Build history of the part. All positions in model axes, mm. Face numbers are marked on the shaded views. A direction names the side the tool comes from. Give positions to 0.01 mm unless a question says otherwise; leave off trailing zeros. Write each loop counter-clockwise with the first axis right and the second up, starting at its lowest first coordinate (ties: lowest second). Pieces come first, ordered by that corner, then holes.
from build123d import *

# Parameters (mm, degrees)
SB_KIRI_80_X_6_1_DEPTH = 20


with BuildPart() as part:
    # Sketch1 → Sb kiriş 80 X 6(1) (new body)
    with BuildSketch(Plane.YZ):
        with BuildLine():
            Line((-20, -40), (-20, -38.04146021))
            ThreePointArc((-20, -38.04146021), (-19.289071417, -36.102349061), (-17.493231968, -35.082284273))
            Line((-17.493231968, -35.082284273), (-7.013536064, -33.335540874))
            ThreePointArc((-7.013536064, -33.335540874), (-3.421857166, -31.295411298), (-2, -27.417189))
            Line((-2, -27.417189), (-2, 27.417189))
            ThreePointArc((-2, 27.417189), (-3.421857166, 31.295411298), (-7.013536064, 33.335540874))
            Line((-7.013536064, 33.335540874), (-17.493231968, 35.082284273))
            ThreePointArc((-17.493231968, 35.082284273), (-19.289071417, 36.102349061), (-20, 38.04146021))
            Line((-20, 38.04146021), (-20, 40))
            Line((-20, 40), (20, 40))
            Line((20, 40), (20, 38.04146021))
            ThreePointArc((20, 38.04146021), (19.289071417, 36.102349061), (17.493231968, 35.082284273))
            Line((17.493231968, 35.082284273), (7.013536064, 33.335540874))
            ThreePointArc((7.013536064, 33.335540874), (3.421857166, 31.295411298), (2, 27.417189))
            Line((2, 27.417189), (2, -27.417189))
            ThreePointArc((2, -27.417189), (3.421857166, -31.295411298), (7.013536064, -33.335540874))
            Line((7.013536064, -33.335540874), (17.493231968, -35.082284273))
            ThreePointArc((17.493231968, -35.082284273), (19.289071417, -36.102349061), (20, -38.04146021))
            Line((20, -38.04146021), (20, -40))
            Line((20, -40), (-20, -40))
        make_face()
    extrude(amount=SB_KIRI_80_X_6_1_DEPTH)


solid = part.part
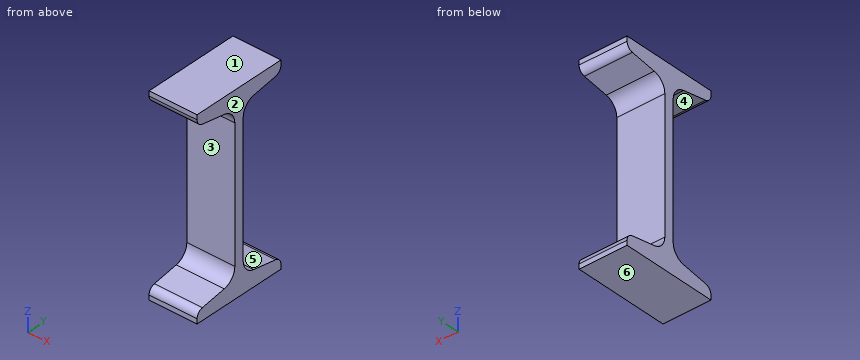
1. Saw through at C-C on y = -13.5. Give the cut face in (x, z).
2. Saw through at D-D on z = 2. Give the cut face in (x, y).
3. 3-axis set-ups, long thin cutter, end or side, ignore diameter. For the marked faces 4, 5 and 6: which of +Z, -Z, +X, -X, +Y, -Y reach the whole face in a straight line?
4. Drop flat-ended pins along their axis: pin 1 (12 mm diameter, centred on x = 7, z = 9, fed in from +Y); pin 2 (4 mm diameter, centred on x = 14.5, z = 30.5, fed in from +Y); pin 3 (6 mm diameter, centred on x = 11.5, z = 3, fed in from -Y). Give the stop position or say it passes through.
5. Saw through at B-B on x = 6.75. Give the cut face in (y, z).
6. Drill centre lines: line 1 along Y through (x, z) = (7.25, 12.5); line 2 along Z through (x, y) = (13.75, -5); line 3 along Z through (x, y) = (5, -10). Where is each one in solid material? Low to high.
7. Saw through at A-A on y = 5.5. Give the cut face in (x, z).
8. Mould opens along Z. For the marked faces 1, 2 and 3 say: pulls with the +Z half, pulls with the -Z half, needs draft (parallel to the pull), parting line crosses it, or undercut.
Outcome:
1. outline: (0, -40) - (20, -40) - (20, -34.42) - (0, -34.42) - close; (0, 34.42) - (20, 34.42) - (20, 40) - (0, 40) - close
2. outline: (0, -2) - (20, -2) - (20, 2) - (0, 2) - close
3. face 4: +X, -X, -Y
3. face 5: +X, -X, +Y
3. face 6: -Z, +X, -X, +Y, -Y
4. pin 1: stops at y = 2
4. pin 2: stops at y = 4.81
4. pin 3: stops at y = -2
5. outline: (-20, -40) - (20, -40) - (20, -38.04) arc R3 ccw to (17.49, -35.08) - (7.01, -33.34) arc R6 cw to (2, -27.42) - (2, 27.42) arc R6 cw to (7.01, 33.34) - (17.49, 35.08) arc R3 ccw to (20, 38.04) - (20, 40) - (-20, 40) - (-20, 38.04) arc R3 ccw to (-17.49, 35.08) - (-7.01, 33.34) arc R6 cw to (-2, 27.42) - (-2, -27.42) arc R6 cw to (-7.01, -33.34) - (-17.49, -35.08) arc R3 ccw to (-20, -38.04) - close
6. line 1: y = -2 to 2
6. line 2: z = -40 to -32.61, 32.61 to 40
6. line 3: z = -40 to -33.83, 33.83 to 40
7. outline: (0, -40) - (20, -40) - (20, -32.87) - (0, -32.87) - close; (0, 32.87) - (20, 32.87) - (20, 40) - (0, 40) - close
8. face 1: pulls with the +Z half
8. face 2: needs draft
8. face 3: undercut
